```python
from build123d import *

# Parameters (mm, degrees)
SKETCH1_R               = 12.7
SKETCH1_R_2             = 7.62
BOSS_EXTRUDE1_DEPTH     = 260.35
SKETCH2_R               = 7.62
BOSS_EXTRUDE2_DEPTH     = 6.35
SKETCH3_R               = 2.2479
CUT_EXTRUDE1_DEPTH      = 1
CUT_EXTRUDE1_DEPTH_BACK = 30.21
SKETCH5_W               = 10.16
SKETCH5_H               = 50.8
SKETCH5_H_2             = 57.15
CUT_EXTRUDE5_DEPTH      = 13.7000001
CUT_EXTRUDE5_DEPTH_BACK = 13.7000001
SKETCH8_W               = 10.16
SKETCH8_H               = 50.8
SKETCH8_H_2             = 57.15
CUT_EXTRUDE6_DEPTH      = 13.7000001
CUT_EXTRUDE6_DEPTH_BACK = 13.7000001
SKETCH7_R               = 3.81
CUT_EXTRUDE4_DEPTH      = 7.3500001


with BuildPart() as part:
    # Sketch1 → Boss-Extrude1 (new body)
    with BuildSketch(Plane(origin=(0, 0, 0), x_dir=(1, 0, 0), z_dir=(0, 1, 0))):
        Circle(SKETCH1_R)
        Circle(SKETCH1_R_2, mode=Mode.SUBTRACT)
    extrude(amount=BOSS_EXTRUDE1_DEPTH)

    # Sketch2 → Boss-Extrude2 (add)
    with BuildSketch(Plane.XZ):
        Circle(SKETCH2_R)
    extrude(amount=-BOSS_EXTRUDE2_DEPTH)

    # Sketch3 → Cut-Extrude1 (cut, two sides)
    with BuildSketch(Plane.XY.offset(16.51)) as cut_extrude1_sk:
        with Locations((0, 101.6)):
            Circle(SKETCH3_R)
    extrude(amount=CUT_EXTRUDE1_DEPTH, mode=Mode.SUBTRACT)
    extrude(cut_extrude1_sk.sketch, amount=-CUT_EXTRUDE1_DEPTH_BACK, mode=Mode.SUBTRACT)

    # Sketch5 → Cut-Extrude5 (cut, two sides)
    with BuildSketch(Plane(origin=(0, 0, 0), x_dir=(0, 0, -1), z_dir=(1, 0, 0))) as cut_extrude5_sk:
        with Locations((0, 38.1)):
            Rectangle(SKETCH5_W, SKETCH5_H)
        with Locations((0, 139.7)):
            Rectangle(SKETCH5_W, SKETCH5_H)
        with Locations((0, 219.075)):
            Rectangle(SKETCH5_W, SKETCH5_H_2)
    extrude(amount=CUT_EXTRUDE5_DEPTH, mode=Mode.SUBTRACT)
    extrude(cut_extrude5_sk.sketch, amount=-CUT_EXTRUDE5_DEPTH_BACK, mode=Mode.SUBTRACT)

    # Sketch8 → Cut-Extrude6 (cut, two sides)
    with BuildSketch(Plane.XY) as cut_extrude6_sk:
        with Locations((0, 38.1)):
            Rectangle(SKETCH8_W, SKETCH8_H)
        with Locations((0, 139.7)):
            Rectangle(SKETCH8_W, SKETCH8_H)
        with Locations((0, 219.075)):
            Rectangle(SKETCH8_W, SKETCH8_H_2)
    extrude(amount=CUT_EXTRUDE6_DEPTH, mode=Mode.SUBTRACT)
    extrude(cut_extrude6_sk.sketch, amount=-CUT_EXTRUDE6_DEPTH_BACK, mode=Mode.SUBTRACT)

    # Sketch7 → Cut-Extrude4 (cut, through all)
    with BuildSketch(Plane(origin=(0, 6.35, 0), x_dir=(1, 0, 0), z_dir=(0, 1, 0))):
        Circle(SKETCH7_R)
    extrude(amount=-CUT_EXTRUDE4_DEPTH, mode=Mode.SUBTRACT)


solid = part.part
```
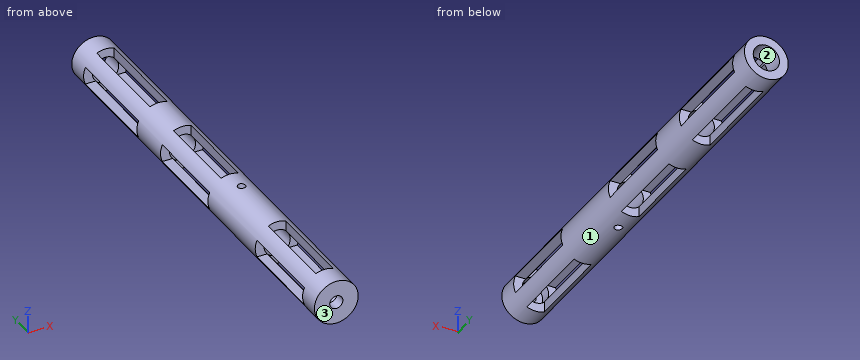
The model under review builds one solid part; all positions refer to its coordinate system, in mm. Face numbers are marked on the shaded views. Round coordinates to 2 decimals unless told otherwise and drop trailing zeros. Loops run counter-clockwise (first coordinate to the right, second up) from the corner with the lowest first, then second, coordinate; pieces in that order, holes last. Notation, with made-up numbers: M -37.75,34 L -27.75,34 A14 ccw -27.75,42 Z; hole C 65,13 d10. An arc over 180 degrees is marked long. Answer as a JSON object with one key per item and string values.
(1) Take a section at B-B on y = 101.6. Give the boundary of the cut face in (x, z), and give its area (3 significant figures).
Resolved:
{"outline": "M -2.25,-12.5 L -2.25,-7.28 A7.62 cw -2.25,7.28 L -2.25,12.5 A12.7 ccw Z; M 2.25,-12.5 A12.7 ccw 2.25,12.5 L 2.25,7.28 A7.62 cw 2.25,-7.28 Z", "area": "278 mm²"}
(2) Clearance check with flat-ended pins moving along their axes: P1, Ø6.5, axis at y = 44.5, z = -8.5, coming from the +X side; P2, Ø1.5, axis at x = 4, y = 137, coming from the -Z side; P3, Ø5, axis at y = 145.5, z = 8.5, coming from the +X side; P4, Ø2, axis at y = 89, z = 9.5, coming from the -X side. State where each tip first meets the part, or that it passes through.
Resolved:
{"P1": "x = 11.56", "P2": "through", "P3": "x = 11.19", "P4": "x = -9.44"}
(3) To check wall thickness, follow line 1 along Y through (x, z) = (7.25, 2.5); line 2 along Y through (x, z) = (0, 9.05); line 3 along Z through (x, y) = (0, 2.25). State the ranges of each line that lie inside material, in increasing order.
Resolved:
{"line 1": "0 to 12.7, 63.5 to 114.3, 165.1 to 190.5, 247.65 to 260.35", "line 2": "0 to 12.7, 63.5 to 99.35, 103.85 to 114.3, 165.1 to 190.5, 247.65 to 260.35", "line 3": "-12.7 to -3.81, 3.81 to 12.7"}
(4) Take a section at A-A on y = 33. Give the boundary of the cut face in (x, z).
Resolved:
{"outline": "M -11.64,-5.08 A12.7 ccw -5.08,-11.64 L -5.08,-5.68 A7.62 cw -5.68,-5.08 Z; M -11.64,5.08 L -5.68,5.08 A7.62 cw -5.08,5.68 L -5.08,11.64 A12.7 ccw Z; M 5.08,-11.64 A12.7 ccw 11.64,-5.08 L 5.68,-5.08 A7.62 cw 5.08,-5.68 Z; M 5.08,5.68 A7.62 cw 5.68,5.08 L 11.64,5.08 A12.7 ccw 5.08,11.64 Z"}
(5) Take a section at C-C on x = 0. Count the separate pieces of the cut face and the enclosed holes in it, and give its area (3 significant figures).
Resolved:
{"separate pieces": "10", "enclosed holes": "0", "area": "1,030 mm²"}
(6) Draft analysis for pull direction X (two halves, no side actions). For the marked faces 1, 2 and 3, state which applies: released by +X, released by -X, zero draft, split by the parting line, or undercut.
Resolved:
{"face 1": "split by the parting line", "face 2": "undercut", "face 3": "zero draft"}
